Autodesk Inventor part; units mm, degrees
ref_plane "YZ Plane" through (0, 0, 0) normal (1, 0, 0) x (0, 1, 0)
ref_plane "XZ Plane" through (0, 0, 0) normal (0, 1, 0) x (-1, 0, 0)
ref_plane "XY Plane" through (0, 0, 0) normal (0, 0, 1) x (1, 0, 0)
sketch "Sketch1" plane through (0, 0, 0) normal (0, 1, 0) x (-1, 0, 0)
  line L0 (0, 0) -> (40.5, 0)
  line L1 (40.5, 0) -> (40.5, -87.5)
  line L2 (40.5, -87.5) -> (0, -87.5)
  line L3 (0, -87.5) -> (0, 0)
  dimension "d0" = 40.5
  dimension "d1" = 87.5
extrude "Extrusion1" add sketch "Sketch1" along normal blind 2
sketch "Sketch3" plane through (0, 2, 0) normal (0, 1, 0) x (1, 0, 0)
  line L0 (-40.5, 0) -> (0, 0)
  line L1 (-40.5, 0) -> (-34.5, 0)
  line L2 (-34.5, 0) -> (-34.5, 6)
  line L3 (-34.5, 6) -> (-40.5, 6)
  line L4 (-40.5, 6) -> (-40.5, 0)
  circle A0 centre (-34.5, 6) radius 3
  line L5 (-40.5, 87.5) -> (-40.5, 0)
  line L6 (-40.5, 87.5) -> (-34.5, 87.5)
  line L7 (-34.5, 87.5) -> (-34.5, 81.5)
  line L8 (-34.5, 81.5) -> (-40.5, 81.5)
  line L9 (-40.5, 81.5) -> (-40.5, 87.5)
  circle A1 centre (-34.5, 81.5) radius 3
  line L10 (0, 0) -> (0, 87.5)
  line L11 (0, 87.5) -> (-6, 87.5)
  line L12 (-6, 87.5) -> (-6, 81.5)
  line L13 (-6, 81.5) -> (0, 81.5)
  line L14 (0, 81.5) -> (0, 87.5)
  circle A2 centre (-6, 81.5) radius 3
  dimension "d4" = 6
  dimension "d5" = 6
  dimension "d6" = 6
  dimension "d7" = 6
  dimension "d8" = 6
  dimension "d9" = 6
  dimension "d10" = 6
  dimension "d11" = 6
  dimension "d12" = 6
extrude "Extrusion2" add sketch "Sketch3" along normal blind 23 contours A0 L3 L2 | L2 L3 A0 | A1 L7 L8 | L8 L7 A1 | A2 L12 L13 | L13 L12 A2
sketch "Sketch4" plane through (-34.5, 25, -6) normal (0, 1, 0) x (1, 0, 0)
  circle A0 centre (0, 0) radius 1.5
  point P0 (34.5, -6)
  dimension "d15" = 3
sketch "Sketch5" plane through (-34.5, 25, -81.5) normal (0, 1, 0) x (1, 0, 0)
  circle A0 centre (0, 0) radius 1.5
  point P0 (34.5, -81.5)
  dimension "d16" = 3
sketch "Sketch6" plane through (-6, 25, -81.5) normal (0, 1, 0) x (1, 0, 0)
  circle A0 centre (0, 0) radius 1.5
  point P0 (6, -81.5)
  dimension "d17" = 3
extrude "Extrusion3" cut sketch "Sketch4" against normal blind 12
extrude "Extrusion4" cut sketch "Sketch5" against normal blind 12
extrude "Extrusion5" cut sketch "Sketch6" against normal blind 12
sketch "Sketch7" plane through (0, 0, 0) normal (0, -1, 0) x (1, 0, 0)
  line L0 (0, 0) -> (0, -87.5)
  line L1 (0, 0) -> (2, 0)
  line L2 (2, 0) -> (2, -87.5)
  line L3 (2, -87.5) -> (0, -87.5)
  line L4 (0, -87.5) -> (0, 0)
  line L5 (-40.5, 0) -> (0, 0)
  line L6 (-40.5, 0) -> (-42.5, 0)
  line L7 (-42.5, 0) -> (-42.5, -87.5)
  line L8 (-42.5, -87.5) -> (-40.5, -87.5)
  line L9 (-40.5, -87.5) -> (-40.5, 0)
  line L10 (-42.5, -87.5) -> (2, -87.5)
  line L11 (2, -87.5) -> (2, -89.5)
  line L12 (2, -89.5) -> (-42.5, -89.5)
  line L13 (-42.5, -89.5) -> (-42.5, -87.5)
  line L14 (-42.5, 0) -> (2, 0)
  line L15 (2, 0) -> (2, 2)
  line L16 (2, 2) -> (-42.5, 2)
  line L17 (-42.5, 2) -> (-42.5, 0)
  dimension "d24" = 2
  dimension "d25" = 2
  dimension "d26" = 2
  dimension "d27" = 2
extrude "Extrusion6" add sketch "Sketch7" against normal blind 27 contours L1 L2 L3 L0 | L5 L6 L17 L16 L15 L1 | L3 L11 L12 L13 L8 L10 | L9 L8 L7 L6
fillet "Fillet1" radius 4 8 edges at (2, 13.5, 2) (2, 13.5, -89.5) (-42.5, 13.5, -89.5) (-42.5, 13.5, 2) (-20.25, 0, 2) (-42.5, 0, -43.75) (-20.25, 0, -89.5) (2, 0, -43.75)
properties part number "BottomcaseV2"
Input: part model. Units: mm. Frame: model coordinates. A direction names the side the tool comes from. Give positions to 0.01 mm unless a question says otherwise; leave off trailing zeros. Order: outer loops, then holes, each group sorted by start corner. A loop starts at its lowest first (then second) coordinate and runs counter-clockwise, first axis right, second up. Notation, with made-up numbers: (41, 40.5) - (66, 40.5) arc R16 cw to (66, 63.5) - close; hole circle Ø5 at (71, 22). An arc over 180 degrees is marked (long way). Answer as a JSON object with one key per item and string values. Group by question number.
Q1. Cut plane A-A, the plane y = 18.25. Output: boundary loops of the cut face in (x, z).
Q2. Mould query, pull axis X, two halves, no side actions, for faces 3 (the face through (-20, 15, -89.5)), 4 (the face through (0.797, 15.661, 0.859)), 5 (the face through (-37.5, 13.3, -5.9)). Classes: pulls with the +X half, pulls with the -X half, needs draft (parallel to the pull), parting line crosses it, or undercut.
Q3. Cut plane C-C, the plane z = -81.5. Output: boundary loops of the cut face in (x, y), then the cut area to 3 significant figures.
Q4. Line query: probe 1 along Z at (x, y) = (-6, 17); probe 2 along Z at (x, y) = (-34.5, 16.5); probe 3 along X at (y, z) = (20.5, -6). Output: solid intervals per line, ascending.
Q5. Cut plane D-D, the plane x = -34.5. Output: boundary loops of the cut face in (y, z).
Q6. Cut plane B-B, the plane y = 6.5. Output: boundary loops of the cut face in (x, z).
Q7. First-contact query: pin 1 Ø3 at (x, z) = (-34.5, -80) entering from +Y; pin 2 Ø12 at (x, z) = (-22.5, -37) entering from +Y; pin 3 Ø5 at (x, z) = (-6, -81.5) entering from -Y; pin 4 Ø0.9 at (x, z) = (-5.5, -81.5) entering from +Y. Flat tips, straight axial feed; report the tip coordinate or a pass-through.
Q8. Set-up query: faces 1 (the face through (-35, 13, -6)), 2 (the face through (-20, 0, -43)). Return all of +Z, -Z, +X, -X, +Y, -Y with unobstructed straight access to the full face (end or side cutting, diameter ignored); none if empty.
Results:
{
 "1": {"outline": "(-42.5, -85.5) arc R4 ccw to (-38.5, -89.5) - (-2, -89.5) arc R4 ccw to (2, -85.5) - (2, -2) arc R4 ccw to (-2, 2) - (-38.5, 2) arc R4 ccw to (-42.5, -2) - close; circle Ø6 at (-34.5, -81.5); circle Ø6 at (-34.5, -6); circle Ø6 at (-6, -81.5); hole (-40.5, -87.5) - (0, -87.5) - (0, 0) - (-40.5, 0) - close; hole circle Ø3 at (-34.5, -81.5); hole circle Ø3 at (-34.5, -6); hole circle Ø3 at (-6, -81.5)"},
 "2": {"face 3": "needs draft", "face 4": "pulls with the +X half", "face 5": "undercut"},
 "3": {"outline": "(-42.5, 4) arc R4 ccw to (-38.5, 0) - (-2, 0) arc R4 ccw to (2, 4) - (2, 27) - (0, 27) - (0, 2) - (-3, 2) - (-3, 25) - (-4.5, 25) - (-4.5, 13) - (-7.5, 13) - (-7.5, 25) - (-9, 25) - (-9, 2) - (-31.5, 2) - (-31.5, 25) - (-33, 25) - (-33, 13) - (-36, 13) - (-36, 25) - (-37.5, 25) - (-37.5, 2) - (-40.5, 2) - (-40.5, 27) - (-42.5, 27) - close", "area": "386 mm^2"},
 "4": {"probe 1": "-89.5 to -87.5, -84.5 to -83, -80 to -78.5, 0 to 2", "probe 2": "-89.5 to -87.5, -84.5 to -83, -80 to -78.5, -9 to -7.5, -4.5 to -3, 0 to 2", "probe 3": "-42.5 to -40.5, -37.5 to -36, -33 to -31.5, 0 to 2"},
 "5": {"outline": "(0, -85.5) arc R4 ccw to (4, -89.5) - (27, -89.5) - (27, -87.5) - (2, -87.5) - (2, -84.5) - (25, -84.5) - (25, -83) - (13, -83) - (13, -80) - (25, -80) - (25, -78.5) - (2, -78.5) - (2, -9) - (25, -9) - (25, -7.5) - (13, -7.5) - (13, -4.5) - (25, -4.5) - (25, -3) - (2, -3) - (2, 0) - (27, 0) - (27, 2) - (4, 2) arc R4 ccw to (0, -2) - close"},
 "6": {"outline": "(-42.5, -85.5) arc R4 ccw to (-38.5, -89.5) - (-2, -89.5) arc R4 ccw to (2, -85.5) - (2, -2) arc R4 ccw to (-2, 2) - (-38.5, 2) arc R4 ccw to (-42.5, -2) - close; circle Ø6 at (-34.5, -81.5); circle Ø6 at (-34.5, -6); circle Ø6 at (-6, -81.5); hole (-40.5, -87.5) - (0, -87.5) - (0, 0) - (-40.5, 0) - close"},
 "7": {"pin 1": "y = 25", "pin 2": "y = 2", "pin 3": "y = 0", "pin 4": "y = 13"},
 "8": {"face 1": "+Y", "face 2": "+Z, -Z, +X, -X, -Y"}
}
